from build123d import *

# Parameters (mm, degrees)
F0_W     = 415
F0_H     = 670
F1_DEPTH = 25
F2_T     = -20
F3_R     = 4
F4_DEPTH = 5


with BuildPart() as f1:
    # F0 (on Top) → F1 (new body)
    with BuildSketch(Plane.XY):
        Rectangle(F0_W, F0_H)
    extrude(amount=F1_DEPTH)

    # F2
    f2_openings = [f1.faces().sort_by_distance(p)[0] for p in [
        (0, 0, 0),
    ]]
    offset(amount=F2_T, openings=f2_openings)

    # F3 (on face) → F4 (cut)
    with BuildSketch(Plane(origin=(0, 0, 0), x_dir=(1, 0, 0), z_dir=(0, 0, -1))):
        with Locations((-197.5, 275)):
            Circle(F3_R)
        with Locations((-197.5, 205)):
            Circle(F3_R)
        with Locations((197.5, 275)):
            Circle(F3_R)
        with Locations((197.5, 205)):
            Circle(F3_R)
        with Locations((-147.5, 325)):
            Circle(F3_R)
        with Locations((-77.5, 325)):
            Circle(F3_R)
        with Locations((-77.5, -325)):
            Circle(F3_R)
        with Locations((-147.5, -325)):
            Circle(F3_R)
    extrude(amount=-F4_DEPTH, mode=Mode.SUBTRACT)


solid = f1.part
Design review of the part built by this model. Coordinates are the model's own, in mm. Round coordinates to 2 decimals unless told otherwise and drop trailing zeros. Write each loop counter-clockwise with the first axis right and the second up, starting at its lowest first coordinate (ties: lowest second). Pieces come first, ordered by that corner, then holes. Notation, with made-up numbers: (77.25, 40) - (121.25, 40) arc R9 cw to (121.25, 52) - close; hole circle Ø7 at (-24, 67.25). An arc over 180 degrees is marked (long way). Use a Markdown table: item, result. Add a question column.
1. We need section A-A (x = -123). State the section outline as (y, z) points, then the cut area to 3 significant figures.
2. We need section B-B (y = 243.5). State the section outline as (x, z) points, then the cut area to 3 significant figures.
3. Wall thickness on probe 1 along Y at (x, z) = (-147.5, 3.95); probe 2 along X at (y, z) = (-325, 1.6); probe 3 along X at (y, z) = (-205, 2.25): over which ranges is each line inside the solid? List them lowest first.
4. Clearance check with a flat-ended pin moving along its axis: pin 1 (6.5 mm diameter, centred on x = 197.5, y = -275, fed in from -Z). State where the tip first meets the part, or that it passes through.
5. Mouldability with a two-part tool opening along Y and no side actions: class faces 1 (the face through (207.5, -5, 12)), 2 (the face through (-3, -335, 12)), 3 (the face through (-3, 335, 12)), 4 (the face through (-3, 4, 5)) as +Y half, -Y half, draft (parallel to the pull), parting line (faces both ways), or undercut.
Output:
| question | item | result |
|---|---|---|
| 1 | outline | (-335, 0) - (-315, 0) - (-315, 5) - (315, 5) - (315, 0) - (335, 0) - (335, 25) - (-335, 25) - close |
| 1 | area | 13,600 mm2 |
| 2 | outline | (-207.5, 0) - (-187.5, 0) - (-187.5, 5) - (187.5, 5) - (187.5, 0) - (207.5, 0) - (207.5, 25) - (-207.5, 25) - close |
| 2 | area | 8,500 mm2 |
| 3 | probe 1 | y = -335 to -329, -321 to -315, 315 to 321, 329 to 335 |
| 3 | probe 2 | x = -207.5 to -151.5, -143.5 to -81.5, -73.5 to 207.5 |
| 3 | probe 3 | x = -207.5 to -201.5, -193.5 to -187.5, 187.5 to 193.5, 201.5 to 207.5 |
| 4 | pin 1 | stops at z = 5 |
| 5 | face 1 | draft |
| 5 | face 2 | -Y half |
| 5 | face 3 | +Y half |
| 5 | face 4 | undercut |
